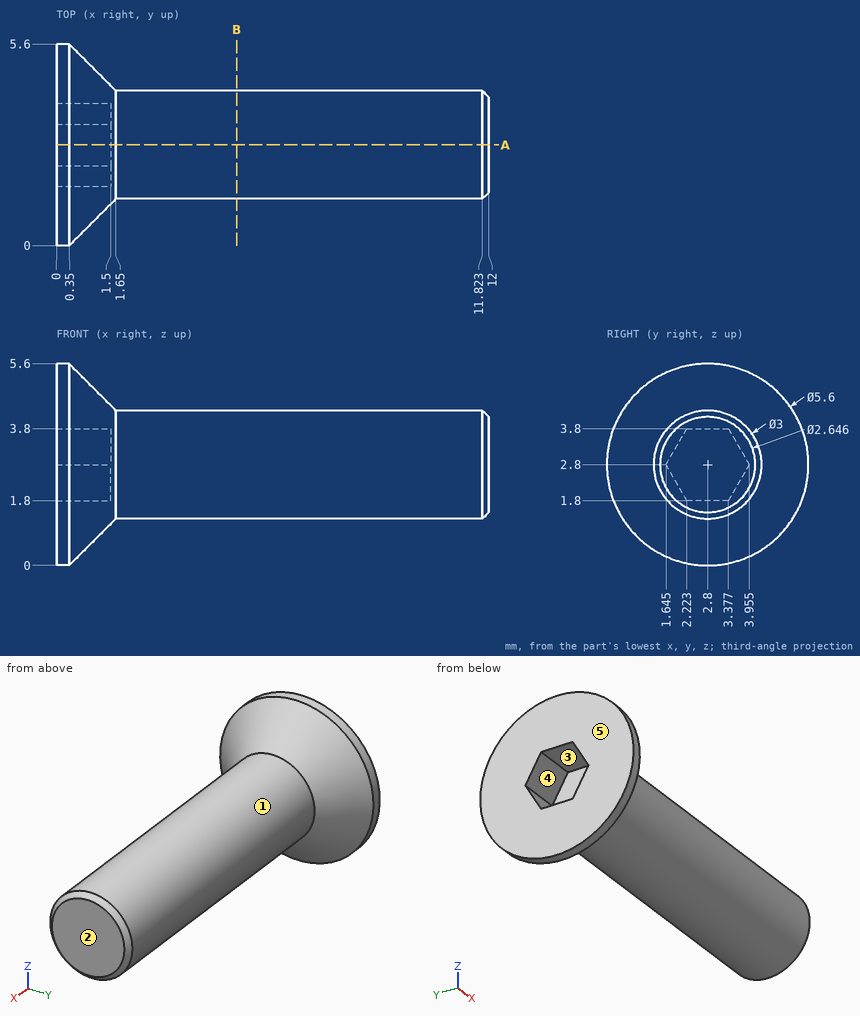
Input: dimensioned drawing with shaded views. Units: mm. Origin: part minimum x, y, z. A direction names the side the tool comes from. Give positions to 0.01 mm unless a question says otherwise; leave off trailing zeros. Write each loop counter-clockwise with the first axis right and the second up, starting at its lowest first coordinate (ties: lowest second). Pieces come first, ordered by that corner, then holes. Notation, with made-up numbers: (83.5, 48.5) - (133.5, 48.5) arc R20 ccw to (133.5, 59.5) - close; hole circle Ø11 at (28.25, -37.75). An arc over 180 degrees is marked (long way). Write item = value, one per line. Start each with the question number.
1) Cut plane A-A (y = 2.8). Return loops of the section in (x, z).
2) Pin query (flat end, axial travel): pin 1 (0.9 mm diameter, centred on x = 1, y = 2.5, fed in from +Z) (1 decimal); pin 2 (3 mm diameter, centred on x = 1.5, z = 1, fed in from -Y). Return the tip coordinate at first contact, or that it passes through.
3) Draft query along Y for the marked faces 1, 2 and 3. Return one class per face: pulls with the +Y half, pulls with the -Y half, needs draft (parallel to the pull), parting line crosses it, or undercut.
4) Reachability of the marked faces 4 and 5 from +Z, -Z, +X, -X, +Y, -Y: full face, straight path, thin tool, end or side. Return the list, or none.
5) Cut plane B-B (x = 5). Return loops of the section in (y, z).
6) Material intervals for L1, parallel to Y at x = 1.25, z = 2.85 (1 decimal); L2, parallel to X at y = 2.7, z = 2.3; L3, parallel to Z at x = 8, y = 2.1 (1 decimal), sorted ascending. Write a range as [from, to].
Answers follow:
q1.outline = (0, 0) - (0.35, 0) - (1.65, 1.3) - (11.82, 1.3) - (12, 1.48) - (12, 4.12) - (11.82, 4.3) - (1.65, 4.3) - (0.35, 5.6) - (0, 5.6) - (0, 3.8) - (1.5, 3.8) - (1.5, 1.8) - (0, 1.8) - close
q2.pin_1 = 5.4
q2.pin_2 = 0.13
q3.face_1 = parting line crosses it
q3.face_2 = needs draft
q3.face_3 = undercut
q4.face_4 = -X
q4.face_5 = +Z, -Z, -X, +Y, -Y
q5.outline = circle Ø3 at (2.8, 2.8)
q6.L1 = [0.9, 1.7], [3.9, 4.7]
q6.L2 = [1.5, 12]
q6.L3 = [1.5, 4.1]
